```python
from build123d import *

# Parameters (mm, degrees)
F0_R     = 15.6
F0_R_2   = 13.1
F1_DEPTH = 25
F1_TAPER = -1
F2_R     = 22.25
F2_R_2   = 12.6635
F3_DEPTH = 3.15
F5_R     = 20.05
F5_R_2   = 17.55
F6_DEPTH = 45
F6_TAPER = -0.75
F7_SIZE  = 1.6109


with BuildPart() as f1:
    # F0 (on Top) → F1 (new body)
    with BuildSketch(Plane.XY):
        Circle(F0_R)
        Circle(F0_R_2, mode=Mode.SUBTRACT)
    extrude(amount=F1_DEPTH, taper=F1_TAPER)

    # F2 (on face) → F3 (join)
    with BuildSketch(Plane.XY.offset(25)):
        Circle(F2_R)
        Circle(F2_R_2, mode=Mode.SUBTRACT)
    extrude(amount=F3_DEPTH)

    # F5 (on offset) → F6 (join, through all)
    with BuildSketch(Plane.XY.offset(73.15)):
        Circle(F5_R)
        Circle(F5_R_2, mode=Mode.SUBTRACT)
    extrude(amount=-F6_DEPTH, taper=F6_TAPER)

    # F7
    f7_edges = [f1.edges().sort_by_distance(p)[0] for p in [
        (-22.25, 0, 28.15),
    ]]
    chamfer(f7_edges, length=F7_SIZE)


solid = f1.part
```
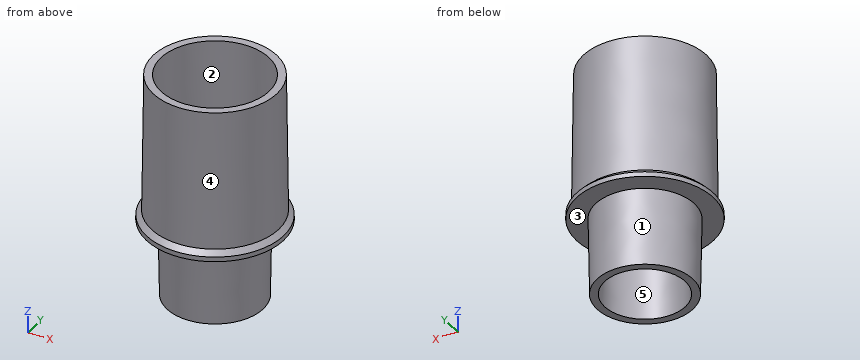
Read the model definition and answer for the solid it produces. Units are mm, in the model's axes. Face numbers are marked on the shaded views. A direction names the side the tool comes from. Coordinates: 2 decimals unless noted, no trailing zeros. Order: outer loops, then holes, each group sorted by start corner. A loop starts at its lowest first (then second) coordinate and runs counter-clockwise, first axis right, second up. Notation, with made-up numbers: (20, -32.75) - (36, -32.75) arc R19 ccw to (36, -0.75) - close; hole circle Ø4 at (-1, -40). An arc over 180 degrees is marked (long way). Answer as a JSON object with one key per item and string values. Group by question number.
Item 1: A tool of negligible diameter and unlimited length cuts with its end or side. For the marked faces 4 and 5, from which of +Z, -Z, +X, -X, +Y, -Y can it reach the whole face along a straight path? Write none if from no direction.
Item 2: Section B-B (z = 56) is taken. Give the vertices of the cut face in (x, y).
Item 3: Consider probe 1 along Z at (x, y) = (-12, 6); probe 2 along X at (y, z) = (-14, 60); probe 3 along X at (y, z) = (9.5, 22). Determine where each line is inside the solid, lowest interval first. Write a range as from..to.
Item 4: The mould has two halves that part along Y. Classify the marked faces 1, 2 and 3: +Y half, -Y half, draft (parallel to the pull), parting line (faces both ways), or undercut.
Item 5: Flat-ended cylindrical pins translate along their axes: P1, Ø8, axis at x = -13, z = 61, coming from the -Y side; P2, Ø1.5, axis at x = -14.5, z = 48.5, coming from the -Y side; P3, Ø1, axis at x = 17.5, z = 53.5, coming from the +Y side; P4, Ø7.5, axis at x = -4, y = -5.5, coming from the -Z side. Find the tip coordinate at first contact, or state that the pin passes through.
Item 6: Section A-A (z = 45.5) is taken. Give the vertices of the cut face in (x, y).
Results are:
{
 "1": {"face 4": "+Z", "face 5": "-Z"},
 "2": {"outline": "circle Ø40.55 at (0, 0); hole circle Ø34.65 at (0, 0)"},
 "3": {"probe 1": "z = 0..28.15", "probe 2": "x = -14.59..-10.3, 10.3..14.59", "probe 3": "x = -12.85..-8.45, 8.45..12.85"},
 "4": {"face 1": "parting line", "face 2": "undercut", "face 3": "draft"},
 "5": {"P1": "stops at y = -18.1", "P2": "stops at y = -15.03", "P3": "stops at y = 11.11", "P4": "passes through"},
 "6": {"outline": "circle Ø40.82 at (0, 0); hole circle Ø34.38 at (0, 0)"}
}
